```python
from build123d import *

# Parameters (mm, degrees)
BOX005_W          = 2.5
BOX005_H          = 6.5
BOX005_DEPTH      = 5
BOX006_W          = 2.5
BOX006_H          = 6.5
BOX006_DEPTH      = 5
BOX007_W          = 2.5
BOX007_H          = 6.5
BOX007_DEPTH      = 5
BOX004_W          = 2.5
BOX004_H          = 6.5
BOX004_DEPTH      = 5
CYLINDER001_R     = 1.4
CYLINDER001_DEPTH = 6.1
CYLINDER002_R     = 1.4
CYLINDER002_DEPTH = 6.1
CYLINDER003_R     = 1.4
CYLINDER003_DEPTH = 6.1
CYLINDER_R        = 1.4
CYLINDER_DEPTH    = 6.1
EXTRUDE_DEPTH     = 7


with BuildPart() as cube001:
    # Box005 → Box005 (new body)
    with BuildSketch(Plane(origin=(-3, 0, 1.8), x_dir=(1, 0, 0), z_dir=(0, 0, 1))):
        with Locations((1.25, 3.25)):
            Rectangle(BOX005_W, BOX005_H)
    extrude(amount=BOX005_DEPTH)


with BuildPart() as cube002:
    # Box006 → Box006 (new body)
    with BuildSketch(Plane(origin=(0.5, 0, 1.8), x_dir=(1, 0, 0), z_dir=(0, 0, 1))):
        with Locations((1.25, 3.25)):
            Rectangle(BOX006_W, BOX006_H)
    extrude(amount=BOX006_DEPTH)


with BuildPart() as cube003:
    # Box007 → Box007 (new body)
    with BuildSketch(Plane(origin=(4, 0, 1.8), x_dir=(1, 0, 0), z_dir=(0, 0, 1))):
        with Locations((1.25, 3.25)):
            Rectangle(BOX007_W, BOX007_H)
    extrude(amount=BOX007_DEPTH)


with BuildPart() as cube:
    # Box004 → Box004 (new body)
    with BuildSketch(Plane(origin=(-6.5, 0, 1.8), x_dir=(1, 0, 0), z_dir=(0, 0, 1))):
        with Locations((1.25, 3.25)):
            Rectangle(BOX004_W, BOX004_H)
    extrude(amount=BOX004_DEPTH)


with BuildPart() as cylinder001:
    # Cylinder001 → Cylinder001 (new body)
    with BuildSketch(Plane(origin=(5.25, 4.1, 6.8), x_dir=(1, 0, 0), z_dir=(0, 0, 1))):
        Circle(CYLINDER001_R)
    extrude(amount=CYLINDER001_DEPTH)


with BuildPart() as cylinder002:
    # Cylinder002 → Cylinder002 (new body)
    with BuildSketch(Plane(origin=(-1.75, 4.1, 6.8), x_dir=(1, 0, 0), z_dir=(0, 0, 1))):
        Circle(CYLINDER002_R)
    extrude(amount=CYLINDER002_DEPTH)


with BuildPart() as cylinder003:
    # Cylinder003 → Cylinder003 (new body)
    with BuildSketch(Plane(origin=(-5.25, 4.1, 6.8), x_dir=(1, 0, 0), z_dir=(0, 0, 1))):
        Circle(CYLINDER003_R)
    extrude(amount=CYLINDER003_DEPTH)


with BuildPart() as cylinder:
    # Cylinder → Cylinder (new body)
    with BuildSketch(Plane(origin=(1.75, 4.1, 6.8), x_dir=(1, 0, 0), z_dir=(0, 0, 1))):
        Circle(CYLINDER_R)
    extrude(amount=CYLINDER_DEPTH)


with BuildPart() as plastic_body:
    # Wire → Extrude (new body, symmetric)
    with BuildSketch(Plane.YZ):
        Polygon((0, 0), (0, 7.4), (2, 12.6), (6.2, 12.6), (7.5, 9), (8.2, 9), (8.2, 0), align=None)
    extrude(amount=EXTRUDE_DEPTH, both=True)

    # Cut: cut Cylinder
    add(cylinder.part, mode=Mode.SUBTRACT)

    # Cut001: cut Cylinder003
    add(cylinder003.part, mode=Mode.SUBTRACT)

    # Cut002: cut Cylinder002
    add(cylinder002.part, mode=Mode.SUBTRACT)

    # Cut003: cut Cylinder001
    add(cylinder001.part, mode=Mode.SUBTRACT)

    # Cut004: cut Cube
    add(cube.part, mode=Mode.SUBTRACT)

    # Cut005: cut Cube003
    add(cube003.part, mode=Mode.SUBTRACT)

    # Cut006: cut Cube002
    add(cube002.part, mode=Mode.SUBTRACT)

    # Cut007: cut Cube001
    add(cube001.part, mode=Mode.SUBTRACT)


solid = plastic_body.part
```
The listing builds one solid part. Answer for the finished solid, in the listing's coordinates (mm). A direction names the side the tool comes from. Coordinates: 2 decimals unless noted, no trailing zeros. Write each loop counter-clockwise with the first axis right and the second up, starting at its lowest first coordinate (ties: lowest second). Pieces come first, ordered by that corner, then holes. Notation, with made-up numbers: (17.5, 50.25) - (54.5, 50.25) arc R20 cw to (54.5, 55.25) - close; hole circle Ø8 at (44.5, 43.25). An arc over 180 degrees is marked (long way). Return JSON: item names as keys, results as strings. Group by question number.
Q1. For a pull along Y with two mould halves and no side action, classify faces 1 (the flat face through (2, 6.5, 4)), 2 (the flat face through (0.1, 6.84, 10.83)), 3 (the flat face through (-5, 3, 1.8)), 4 (the cylindrical face through (-1, 5.28, 9.66)) as +Y half, -Y half, draft (parallel to the pull), parting line (faces both ways), or undercut.
Q2. A flat-ended cylindrical pin translates along its axis: pin 1 Ø2 at (x, y) = (-5.25, 4.1) entering from +Z. Find the tip coordinate at first contact, or state that the pin passes through.
Q3. The part is cut by section C-C on y = 2.5. Write down the section's boundary in (x, z).
Q4. The part is cut by section B-B on z = 7. Write down the section's boundary in (x, y), and give its area (3 significant figures).
Q5. Which of the six approach directions +Z, -Z, +X, -X, +Y, -Y give full straight-line access (tool end or side, diameter ignored) to faces 5 (the flat face through (5, 6.5, 4)), 6 (the flat face through (0, 1, 10)), 7 (the cylindrical face through (6.585, 4.521, 9.659))?
Q6. The part is cut by section A-A on x = -1.75. Write down the section's boundary in (y, z).
Q7. The part is cut by section D-D on x = 3.5. Write down the section's boundary in (y, z), and give its area (3 significant figures).
Q8. Find the intervals of material crossed by line 1 along X through (y, z) = (4.1, 8.55); line 2 along X through (y, z) = (4.75, 3); line 3 along Z through (x, y) = (-0.75, 2.5), in increasing order. Write a range as [from, to].
Evaluation:
{
 "1": {"face 1": "-Y half", "face 2": "+Y half", "face 3": "draft", "face 4": "undercut"},
 "2": {"pin 1": "stops at z = 1.8"},
 "3": {"outline": "(-7, 0) - (7, 0) - (7, 12.6) - (-7, 12.6) - close; hole (-6.5, 1.8) - (-4, 1.8) - (-4, 6.8) - (-6.5, 6.8) - close; hole (-3, 1.8) - (-0.5, 1.8) - (-0.5, 6.8) - (-3, 6.8) - close; hole (0.5, 1.8) - (3, 1.8) - (3, 6.8) - (0.5, 6.8) - close; hole (4, 1.8) - (6.5, 1.8) - (6.5, 6.8) - (4, 6.8) - close"},
 "4": {"outline": "(-7, 0) - (7, 0) - (7, 8.2) - (-7, 8.2) - close; hole circle Ø2.8 at (-5.25, 4.1); hole circle Ø2.8 at (-1.75, 4.1); hole circle Ø2.8 at (1.75, 4.1); hole circle Ø2.8 at (5.25, 4.1)", "area": "90.2 mm2"},
 "5": {"face 5": "-Y", "face 6": "+Z, +X, -X, -Y", "face 7": "+Z"},
 "6": {"outline": "(0, 0) - (8.2, 0) - (8.2, 9) - (7.5, 9) - (6.2, 12.6) - (5.5, 12.6) - (5.5, 6.8) - (6.5, 6.8) - (6.5, 1.8) - (0, 1.8) - close; (0, 6.8) - (2.7, 6.8) - (2.7, 12.6) - (2, 12.6) - (0, 7.4) - close"},
 "7": {"outline": "(0, 0) - (8.2, 0) - (8.2, 9) - (7.5, 9) - (6.2, 12.6) - (2, 12.6) - (0, 7.4) - close", "area": "93.3 mm2"},
 "8": {"line 1": "x = [-7, -6.65], [-3.85, -3.15], [-0.35, 0.35], [3.15, 3.85], [6.65, 7]", "line 2": "x = [-7, -6.5], [-4, -3], [-0.5, 0.5], [3, 4], [6.5, 7]", "line 3": "z = [0, 1.8], [6.8, 12.6]"}
}
